from build123d import *

# Parameters (mm, degrees)
F0_R      = 21.5
F1_DEPTH  = 40
F2_R      = 5
F3_R      = 21.5
F4_DEPTH  = 40
F5_SIZE2  = 7.5
F5_SIZE   = 40
F6_DEPTH  = 10
F7_R      = 10
F10_R     = 4.9
F11_DEPTH = 75
F12_R     = 16.5
F13_DEPTH = 5
F14_R     = 3.1
F15_DEPTH = 85.001
F16_R     = 12.5
F17_DEPTH = 76


with BuildPart() as f1:
    # F0 (on Top) → F1 (new body)
    with BuildSketch(Plane.XY):
        Circle(F0_R)
    extrude(amount=F1_DEPTH)

    # F2
    f2_edges = [f1.edges().sort_by_distance(p)[0] for p in [
        (-21.5, 0, 40),
    ]]
    fillet(f2_edges, radius=F2_R)

    # F3 (on face) → F4 (join)
    with BuildSketch(Plane(origin=(0, 0, 0), x_dir=(1, 0, 0), z_dir=(0, 0, -1))):
        Circle(F3_R)
    extrude(amount=F4_DEPTH)

    # F5
    f5_edges = [f1.edges().sort_by_distance(p)[0] for p in [
        (-21.5, 0, -40),
    ]]
    chamfer(f5_edges, length=F5_SIZE, length2=F5_SIZE2)

    # F6 (add): a face of the model
    f6_faces = [f1.faces().sort_by_distance(p)[0] for p in [
        (0, 0, -40),
    ]]
    extrude(f6_faces, amount=F6_DEPTH)

    # F7
    f7_edges = [f1.edges().sort_by_distance(p)[0] for p in [
        (-21.5, 0, 0),
    ]]
    fillet(f7_edges, radius=F7_R)

    # F8 (on Right) → F9 (revolve, cut)
    with BuildSketch(Plane.YZ):
        Polygon((-7.5, -40.5), (-17.4298945979, -40.5), (-17.4298945979, -47.5), (-17.4298945979, -53.659953177), (-10, -53.659953177), (-10, -47.5), (-7.5, -47.5), align=None)
    revolve(axis=Axis((0, 0, -53.4000843763), (0, 0, -1)), mode=Mode.SUBTRACT)

    # F10 (on face) → F11 (cut)
    with BuildSketch(Plane(origin=(0, 0, -50), x_dir=(1, 0, 0), z_dir=(0, 0, -1))):
        Circle(F10_R)
    extrude(amount=-F11_DEPTH, mode=Mode.SUBTRACT)

    # F12 (on face) → F13 (cut)
    with BuildSketch(Plane.XY.offset(40)):
        Circle(F12_R)
    extrude(amount=-F13_DEPTH, mode=Mode.SUBTRACT)

    # F14 (on face) → F15 (cut, through all)
    with BuildSketch(Plane.XY.offset(35)):
        Circle(F14_R)
    extrude(amount=-F15_DEPTH, mode=Mode.SUBTRACT)

    # F16 (on face) → F17 (cut)
    with BuildSketch(Plane(origin=(0, 0, -50), x_dir=(1, 0, 0), z_dir=(0, 0, -1))):
        Circle(F16_R)
    extrude(amount=-F17_DEPTH, mode=Mode.SUBTRACT)


solid = f1.part
Read the model definition and answer for the solid it produces. Units are mm, in the model's axes. A direction names the side the tool comes from. Coordinates: 2 decimals unless noted, no trailing zeros. Loops run counter-clockwise (first coordinate to the right, second up) from the corner with the lowest first, then second, coordinate; pieces in that order, holes last.
Q1. Each of these flat-tipped pins is pushed along its axis until it touches: pin 1 Ø1 at (x, z) = (10, -28) entering from -Y; pin 2 Ø1 at (y, z) = (-15.5, 19) entering from +X; pin 3 Ø4 at (x, z) = (-14, 24) entering from -Y. Where does it stop, or does it pass through?
Q2. The mould has two halves that part along X. Classify faces 1 (the face through (-11.5, -5.3, -40.5)), 2 (the face through (15.24, -6.32, 37.53)), 3 (the face through (7.752, 14.903, -25.073)): +X half, -X half, draft (parallel to the pull), parting line (faces both ways), or undercut.
Q3. The part is cut by section B-B on z = -27.5. Write down the section's boundary in (x, y).
Q4. The part is cut by section A-A on z = 17.5. Write down the section's boundary in (x, y), and give its area (3 significant figures).
Q5. Which of the six approach directions +Z, -Z, +X, -X, +Y, -Y give full straight-line access (tool end or side, diameter ignored) to faces 4 (the face through (12.932, 5.362, -40.246)), 5 (the face through (-2.799, -21.317, 18.203)), 6 (the face through (-0.2, -3.4, 35))?
Q6. Consider probe 1 along Y at (x, z) = (0, 3.5); probe 2 along Y at (x, z) = (0, 30). Determine where each line is inside the solid, lowest interval first.
Results below:
1. pin 1: stops at y = -13.2
1. pin 2: stops at x = 15.4
1. pin 3: stops at y = -17.84
2. face 1: draft
2. face 2: undercut
2. face 3: parting line
3. outline: circle Ø32.69 at (0, 0); hole circle Ø25 at (0, 0)
4. outline: circle Ø43 at (0, 0); hole circle Ø25 at (0, 0)
4. area: 961 mm2
5. face 4: -Z
5. face 5: +Z, -Z
5. face 6: +Z
6. probe 1: y = -21.5 to -12.5, 12.5 to 21.5
6. probe 2: y = -21.5 to -3.1, 3.1 to 21.5
